Verification items for the finished model (mm, model axes). A direction names the side the tool comes from. Round coordinates to 2 decimals unless told otherwise and drop trailing zeros. Write item = value, one per line. Start each with the question number.
from build123d import *

# Parameters (mm, degrees)
F1_DEPTH = 1
F2_R     = 1
F3_DEPTH = 1.001
F4_R     = 1
F5_DEPTH = 1.001
F6_R     = 1
F7_DEPTH = 1.001


with BuildPart() as f1:
    # F0 (on Front) → F1 (new body)
    with BuildSketch(Plane.XZ):
        Polygon((-18.922574, 24), (-22.922574, 24), (-22.922574, 0), (18.077426, 0), (18.077426, 24), (14.077426, 24), (14.077426, 23), (10.077426, 23), (10.077426, 24), (-14.922574, 24), (-14.922574, 23), (-18.922574, 23), align=None)
    extrude(amount=F1_DEPTH)

    # F2 (on face) → F3 (cut, through all)
    with BuildSketch(Plane.XZ.offset(1)):
        with Locations((-18.436505, 18.492816)):
            Circle(F2_R)
        with Locations((-15.436505, 18.492816)):
            Circle(F2_R)
        with Locations((-12.436505, 18.492816)):
            Circle(F2_R)
        with Locations((-9.436505, 18.492816)):
            Circle(F2_R)
        with Locations((-6.436505, 18.492816)):
            Circle(F2_R)
        with Locations((-3.436505, 18.492816)):
            Circle(F2_R)
        with Locations((-0.436505, 18.492816)):
            Circle(F2_R)
        with Locations((2.563495, 18.492816)):
            Circle(F2_R)
        with Locations((5.563495, 18.492816)):
            Circle(F2_R)
        with Locations((8.563495, 18.492816)):
            Circle(F2_R)
        with Locations((11.563495, 18.492816)):
            Circle(F2_R)
        with Locations((14.563099, 18.541559)):
            Circle(F2_R)
    extrude(amount=-F3_DEPTH, mode=Mode.SUBTRACT)

    # F4 (on face) → F5 (cut, through all)
    with BuildSketch(Plane.XZ.offset(1)):
        with Locations((-17.169001, 15.706128)):
            Circle(F4_R)
        with Locations((-14.169001, 15.706128)):
            Circle(F4_R)
        with Locations((-11.169001, 15.706128)):
            Circle(F4_R)
        with Locations((-8.169001, 15.706128)):
            Circle(F4_R)
        with Locations((-5.169001, 15.706128)):
            Circle(F4_R)
        with Locations((-2.169001, 15.706128)):
            Circle(F4_R)
        with Locations((0.830999, 15.706128)):
            Circle(F4_R)
        with Locations((3.830999, 15.706128)):
            Circle(F4_R)
        with Locations((6.830999, 15.706128)):
            Circle(F4_R)
        with Locations((9.830999, 15.706128)):
            Circle(F4_R)
        with Locations((12.830999, 15.706128)):
            Circle(F4_R)
    extrude(amount=-F5_DEPTH, mode=Mode.SUBTRACT)

    # F6 (on face) → F7 (cut, through all)
    with BuildSketch(Plane.XZ.offset(1)):
        with Locations((-12.836513, 13.417575)):
            Circle(F6_R)
        with Locations((-18.836513, 13.417575)):
            Circle(F6_R)
        with Locations((-15.836513, 13.417575)):
            Circle(F6_R)
        with Locations((-9.836513, 13.417575)):
            Circle(F6_R)
        with Locations((-6.836513, 13.417575)):
            Circle(F6_R)
        with Locations((-3.836513, 13.417575)):
            Circle(F6_R)
        with Locations((-0.836513, 13.417575)):
            Circle(F6_R)
        with Locations((2.163487, 13.417575)):
            Circle(F6_R)
        with Locations((5.163487, 13.417575)):
            Circle(F6_R)
        with Locations((8.163487, 13.417575)):
            Circle(F6_R)
        with Locations((11.163487, 13.417575)):
            Circle(F6_R)
        with Locations((14.163487, 13.417575)):
            Circle(F6_R)
    extrude(amount=-F7_DEPTH, mode=Mode.SUBTRACT)


solid = f1.part
(1) Set-up check for faces 5 (the cylindrical face through (-13.245, -0.507, 15.323)), 6 (the flat face through (12.1, -0.5, 23)): record each of +Z, -Z, +X, -X, +Y, -Y from which the full face is reachable in a straight line by a thin tool's end or side.
(2) Scan lines: line 1 along Z through (x, y) = (-3, -0.05); line 2 along Z through (x, y) = (-13, -0.8); line 3 along Z through (x, y) = (-18.5, -0.5). Record each from-to range of solid material in increasing order. Write a range as from..to.
(3) Draft check along X on faces 1 (the flat face through (18.077, -0.5, 11.8)), 2 (the flat face through (14.077, -0.5, 23.5)), 3 (the cylindrical face through (3.61, -0.51, 14.73)), 4 (the flat face through (-3, -1, 12)). Enter one of: +X half, -X half, draft (parallel to the pull), parting line (faces both ways), or undercut.
(4) Depth check by flat-ended pin: pin 1 (1.6 mm diameter, centred on x = -9.44, z = 18.49, fed in from +Y). Enter the tip coordinate at first touch or a pass-through.
(5) Cross-section at A-A (y = -0.65). Give the number of separate pieces and of enclosed holes in the cut face, and give its area (3 significant figures).
Outcome:
q1.face_5 = +Y, -Y
q1.face_6 = +Z, +Y, -Y
q2.line_1 = 0..12.87, 13.97..15.15, 16.26..17.59, 19.39..24
q2.line_2 = 0..12.43, 14.4..17.67, 19.32..24
q2.line_3 = 0..12.48, 14.36..17.49, 19.49..23
q3.face_1 = +X half
q3.face_2 = undercut
q3.face_3 = undercut
q3.face_4 = draft
q4.pin_1 = through
q5.separate_pieces = 1
q5.enclosed_holes = 35
q5.area = 866 mm^2
